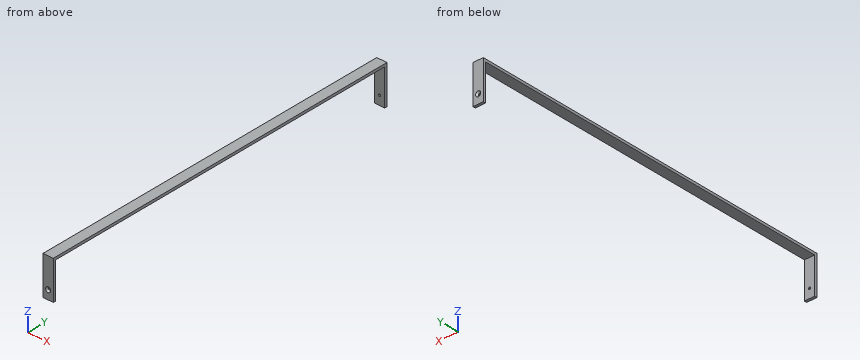
from build123d import *

# Parameters (mm, degrees)
F1_DEPTH       = 20
F3_D           = 8.5
F3_DEPTH       = 15
F3_CSINK_D     = 20
F3_CSINK_ANGLE = 90
F3_TIP         = 2.5536576309


# Not quite as in the source:
# - a pattern or mirror of a feature is missing from the dataset's text; its kind, count and spacing are read off the source's solid


with BuildPart() as f1:
    # F0 (on Right) → F1 (new body, symmetric)
    with BuildSketch(Plane.YZ):
        Polygon((720, 0), (0, 0), (-720, 0), (-720, -150), (-710, -150), (-710, -10), (0, -10), (710, -10), (710, -150), (720, -150), align=None)
    extrude(amount=F1_DEPTH, both=True)

    # F3
    with Locations(Plane.XZ.offset(720)):
        with Locations((0, -115)):
            f3 = CounterSinkHole(F3_D / 2, F3_CSINK_D / 2, depth=F3_DEPTH, counter_sink_angle=F3_CSINK_ANGLE)
            with Locations((0, 0, -(F3_DEPTH + F3_TIP / 2))):  # 118° drill point
                Cone(0, F3_D / 2, F3_TIP, mode=Mode.SUBTRACT)

    # F3_copies: F3 across plane
    add(f3.mirror(Plane.ZX), mode=Mode.SUBTRACT)


solid = f1.part
Input: part model. Units: mm. Frame: model coordinates. Round coordinates to 2 decimals unless told otherwise and drop trailing zeros. Order: outer loops, then holes, each group sorted by start corner. A loop starts at its lowest first (then second) coordinate and runs counter-clockwise, first axis right, second up. Notation, with made-up numbers: (49, 89) - (103, 89) arc R26 cw to (103, 108) - close; hole circle Ø6 at (76.25, 62.5). An arc over 180 degrees is marked (long way). Answer as a JSON object with one key per item and string values. Group by question number.
(1) Cut plane B-B (y = 315). Return loops of the section in (x, z).
(2) Material intervals for probe 1 along Y at (x, z) = (9, -40); probe 2 along X at (y, z) = (-710.85, -115); probe 3 along Z at (x, y) = (0, 712), sorted ascending. Write a range as from..to.
(3) Pin query (flat end, axial travel): P1, Ø11, axis at x = 0, z = -115, coming from the +Y side; P2, Ø13.5, axis at x = 0, z = -115, coming from the +Y side. Return the tip coordinate at first contact, or that it passes through.
(4) Cut plane A-A (z = -62). Return loops of the section in (x, y).
Here are the results:
{
 "1": {"outline": "(-20, -10) - (20, -10) - (20, 0) - (-20, 0) - close"},
 "2": {"probe 1": "y = -720..-710, 710..720", "probe 2": "x = -20..-4.25, 4.25..20", "probe 3": "z = -150..-119.25, -110.75..0"},
 "3": {"P1": "stops at y = 715.5", "P2": "stops at y = 716.75"},
 "4": {"outline": "(-20, -720) - (20, -720) - (20, -710) - (-20, -710) - close; (-20, 710) - (20, 710) - (20, 720) - (-20, 720) - close"}
}
